Source: CAD feature listing. Evaluate the final solid. Frame: model axes, mm. Face numbers are marked on the shaded views. A direction names the side the tool comes from. Coordinates: 2 decimals unless noted, no trailing zeros. Order: outer loops, then holes, each group sorted by start corner. A loop starts at its lowest first (then second) coordinate and runs counter-clockwise, first axis right, second up.
Item 1: Mould query, pull axis X, two halves, no side actions, for the marked faces 1, 2, 3 and 4. Classes: released by +X, released by -X, zero draft, split by the parting line, or undercut.
Item 2: Section C-C on z = 13. Return the cut outline in (x, y), then the cut area to 3 significant figures.
Item 3: Section A-A on y = 29. Return the cut outline in (x, z), then the cut area to 3 significant figures.
Item 4: Section B-B on x = 24.5. Return the cut outline in (y, z).
Item 5: Ray query, line 1 (X direction, y = 28, z = 10); line 2 (Z direction, x = 21, y = 56.5); line 3 (Y direction, x = 7.5, z = 18.75). Return the intervals inside material, ascending.
Item 6: Section D-D on z = 23.25. Return the cut outline in (x, y), then the cut area to 3 significant figures.
Item 7: Reachability of the marked faces 5 and 6 from +Z, -Z, +X, -X, +Y, -Y: full face, straight path, thin tool, end or side. Return the list, or none.
Item 8: Contact query for flat-ended pins moving along their axis: P1, Ø3, axis at x = 36, y = 34, coming from the +Z side; P2, Ø5, axis at x = 5, z = 14.5, coming from the +Y side. Output: stop coordinate, or through.
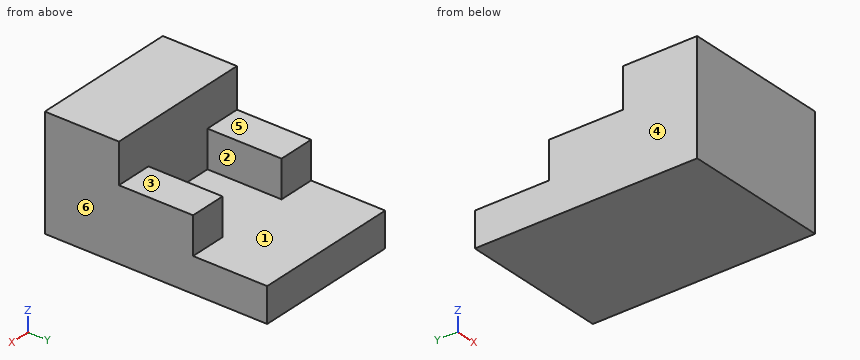
from build123d import *

# Parameters (mm, degrees)
F1_DEPTH = 40
F2_W     = 10
F2_H     = 20
F3_DEPTH = 10


with BuildPart() as f1:
    # F0 (on Right) → F1 (new body)
    with BuildSketch(Plane.YZ):
        Polygon((0, 30), (0, 0), (60, 0), (60, 9.296588), (50, 9.296588), (20, 9.296588), (20, 30), align=None)
    extrude(amount=F1_DEPTH)

    # F2 (on face) → F3 (join)
    with BuildSketch(Plane.XY.offset(9.296588)):
        with Locations((35, 30)):
            Rectangle(F2_W, F2_H)
        with Locations((5, 30)):
            Rectangle(F2_W, F2_H)
    extrude(amount=F3_DEPTH)


solid = f1.part
Answer list:
1. face 1: undercut
1. face 2: undercut
1. face 3: zero draft
1. face 4: released by -X
2. outline: (0, 0) - (40, 0) - (40, 40) - (30, 40) - (30, 20) - (10, 20) - (10, 40) - (0, 40) - close
2. area: 1,200 mm2
3. outline: (0, 0) - (40, 0) - (40, 19.3) - (30, 19.3) - (30, 9.3) - (10, 9.3) - (10, 19.3) - (0, 19.3) - close
3. area: 572 mm2
4. outline: (0, 0) - (60, 0) - (60, 9.3) - (20, 9.3) - (20, 30) - (0, 30) - close
5. line 1: x = 0 to 10, 30 to 40
5. line 2: z = 0 to 9.3
5. line 3: y = 0 to 40
6. outline: (0, 0) - (40, 0) - (40, 20) - (0, 20) - close
6. area: 800 mm2
7. face 5: +Z, +X, -X, +Y
7. face 6: +Z, -Z, +X, +Y, -Y
8. P1: stops at z = 19.3
8. P2: stops at y = 40
